```python
from build123d import *

# Parameters (mm, degrees)
F0_R     = 45.9994
F0_R_2   = 7.53999
F0_R_3   = 2.0955
F1_DEPTH = 25.4
F2_SIZE  = 2.54
F3_SIZE  = 2.54
F4_SIZE  = 2.54


with BuildPart() as f1:
    # F0 (on Front) → F1 (new body)
    with BuildSketch(Plane.XZ):
        Circle(F0_R)
        with Locations((-30.59789, -17.6657)):
            Circle(F0_R_2, mode=Mode.SUBTRACT)
        with Locations((0, -35.3314)):
            Circle(F0_R_3, mode=Mode.SUBTRACT)
        with Locations((30.59789, -17.6657)):
            Circle(F0_R_2, mode=Mode.SUBTRACT)
        with Locations((-30.59789, 17.6657)):
            Circle(F0_R_3, mode=Mode.SUBTRACT)
        with Locations((30.59789, 17.6657)):
            Circle(F0_R_3, mode=Mode.SUBTRACT)
        with Locations((0, 35.3314)):
            Circle(F0_R_2, mode=Mode.SUBTRACT)
    extrude(amount=-F1_DEPTH)

    # F2
    f2_edges = [f1.edges().sort_by_distance(p)[0] for p in [
        (-32.69339, 0, 17.6657),
    ]]
    chamfer(f2_edges, length=F2_SIZE)

    # F3
    f3_edges = [f1.edges().sort_by_distance(p)[0] for p in [
        (28.50239, 0, 17.6657),
    ]]
    chamfer(f3_edges, length=F3_SIZE)

    # F4
    f4_edges = [f1.edges().sort_by_distance(p)[0] for p in [
        (-2.0955, 0, -35.3314),
    ]]
    chamfer(f4_edges, length=F4_SIZE)


solid = f1.part
```
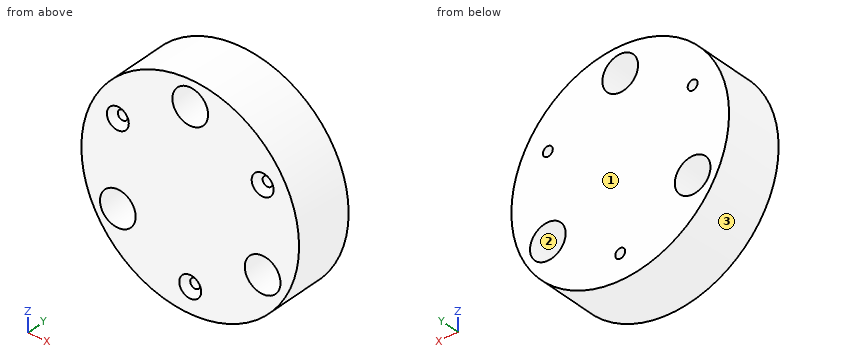
Work out the finished part from the listing and answer in its coordinate system (mm). Face numbers are marked on the shaded views. Give positions to 0.01 mm unless a question says otherwise; leave off trailing zeros. Order: outer loops, then holes, each group sorted by start corner. A loop starts at its lowest first (then second) coordinate and runs counter-clockwise, first axis right, second up.
1. Section C-C, the plane z = -13 is taken. Determine the outline of the cut face in (x, y).
Result sheet:
outline: (-44.12, 0) - (-36.52, 0) - (-36.52, 25.4) - (-44.12, 25.4) - close; (-24.67, 0) - (24.67, 0) - (24.67, 25.4) - (-24.67, 25.4) - close; (36.52, 0) - (44.12, 0) - (44.12, 25.4) - (36.52, 25.4) - close
2. The mould has two halves that part along X. Classify the marked faces 1, 2 and 3: released by +X, released by -X, zero draft, split by the parting line, or undercut.
Result sheet:
face 1: zero draft
face 2: undercut
face 3: split by the parting line
3. Section A-A, the plane x = 0 is taken. Determine the outline of the cut face in (y, z).
Result sheet:
outline: (0, -46) - (25.4, -46) - (25.4, -37.43) - (2.54, -37.43) - (0, -39.97) - close; (0, -30.7) - (2.54, -33.24) - (25.4, -33.24) - (25.4, 27.79) - (0, 27.79) - close; (0, 42.87) - (25.4, 42.87) - (25.4, 46) - (0, 46) - close
4. Section D-D, the plane x = -15 is taken. Determine the outline of the cut face in (y, z) (3 decimals), and give its area (3 significant figures).
Result sheet:
outline: (0, -43.485) - (25.4, -43.485) - (25.4, 43.485) - (0, 43.485) - close
area: 2,210 mm2
5. Section B-B, the plane y = 11.5 is taken. Determine the outline of the cut face in (x, z).
Result sheet:
outline: circle Ø92 at (0, 0); hole circle Ø15.08 at (-30.6, -17.67); hole circle Ø4.19 at (-30.6, 17.67); hole circle Ø15.08 at (0, 35.33); hole circle Ø4.19 at (0, -35.33); hole circle Ø15.08 at (30.6, -17.67); hole circle Ø4.19 at (30.6, 17.67)
6. Straight lines are drawn through the part: L1, parallel to Z at x = 0, y = 18.25; L2, parallel to X at y = 11.75, z = -24; L3, parallel to X at y = 22.25, z = 19.5. For each, find the intervals that lie inside material, in ascending order.
Result sheet:
L1: z = -46 to -37.43, -33.24 to 27.79, 42.87 to 46
L2: x = -39.24 to -34.69, -26.51 to 26.51, 34.69 to 39.24
L3: x = -41.66 to -31.61, -29.58 to 29.58, 31.61 to 41.66
7. Each of these flat-tipped pins is pushed along its axis until it touches: P1, Ø5, axis at x = 4.5, y = 20.5, coming from the +Z side; P2, Ø5.5, axis at x = -30.6, z = 17.67, coming from the +Y side; P3, Ø5, axis at x = 28, y = 14.5, coming from the -Z side; P4, Ø3, axis at y = 18.5, z = 23.5, coming from the -X side. Where does it stop, or does it pass through?
Result sheet:
P1: stops at z = 45.96
P2: stops at y = 25.4
P3: stops at z = -38.28
P4: stops at x = -40.4
